```python
from build123d import *

# Parameters (mm, degrees)
F0_R     = 1.6
F0_W     = 21
F0_H     = 55
F1_DEPTH = 15
F2_W     = 22.6258952171
F2_H     = 57.1813471615
F3_DEPTH = 1
F5_DEPTH = 2
F6_SIZE  = 1.99999


# Not quite as in the source:
# - a fillet or chamfer is up to 0.001 mm smaller than in the source, because OpenCascade refuses the exact size


with BuildPart() as f1:
    # F0 (on Top) → F1 (new body)
    with BuildSketch(Plane.XY):
        with BuildLine():
            Line((12.5, -29.5), (12.5, 29.5))
            ThreePointArc((12.5, 29.5), (0, 42), (-12.5, 29.5))
            Line((-12.5, 29.5), (-12.5, -29.5))
            ThreePointArc((-12.5, -29.5), (0, -42), (12.5, -29.5))
        make_face()
        with Locations((-6, -33.5)):
            Circle(F0_R, mode=Mode.SUBTRACT)
        with Locations((6, -33.5)):
            Circle(F0_R, mode=Mode.SUBTRACT)
        with Locations((-6, 33.5)):
            Circle(F0_R, mode=Mode.SUBTRACT)
        Rectangle(F0_W, F0_H, mode=Mode.SUBTRACT)
        with Locations((6, 33.5)):
            Circle(F0_R, mode=Mode.SUBTRACT)
    extrude(amount=F1_DEPTH)

    # F2 (on Top) → F3 (join)
    with BuildSketch(Plane.XY):
        Rectangle(F2_W, F2_H)
    extrude(amount=F3_DEPTH)

    # F4 (on face) → F5 (cut)
    with BuildSketch(Plane.XY.offset(15)):
        with BuildLine():
            ThreePointArc((1.5, 41.909673646), (0, 42), (-1.5, 41.909673646))
            Line((-1.5, 41.909673646), (-1.5, 27.5))
            Line((-1.5, 27.5), (1.5, 27.5))
            Line((1.5, 27.5), (1.5, 41.909673646))
        make_face()
        with BuildLine():
            Line((1.5, -27.5), (-1.5, -27.5))
            Line((-1.5, -27.5), (-1.5, -41.909673646))
            ThreePointArc((-1.5, -41.909673646), (0, -42), (1.5, -41.909673646))
            Line((1.5, -41.909673646), (1.5, -27.5))
        make_face()
    extrude(amount=-F5_DEPTH, mode=Mode.SUBTRACT)

    # F6 (size 2 in the source; OpenCascade refuses exactly that, so slightly less here)
    f6_edges = [f1.edges().sort_by_distance(p)[0] for p in [
        (-1.5, 34.704837, 15),
        (1.5, 34.704837, 15),
        (1.5, -34.704837, 15),
        (-1.5, -34.704837, 15),
    ]]
    chamfer(f6_edges, length=F6_SIZE)


solid = f1.part
```
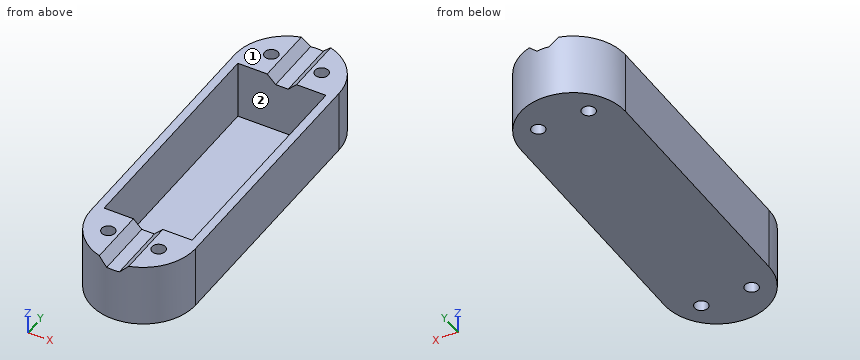
Check sheet for the modelled part. Datum: model origin and axes. Units: mm. Face numbers are marked on the shaded views. A direction names the side the tool comes from. Coordinates: 2 decimals unless noted, no trailing zeros. Order: outer loops, then holes, each group sorted by start corner. A loop starts at its lowest first (then second) coordinate and runs counter-clockwise, first axis right, second up. Notation, with made-up numbers: M 16,66 L 51,66 A17 cw 51,93 Z; hole C 24.5,83.5 d7. An arc over 180 degrees is marked long. One line per question, with ' | ' between items. Start each with the question number.
Item 1: Access from +Z, -Z, +X, -X, +Y, -Y to the whole of each face (thin tool, end or side, straight path). Record for the marked faces 1 and 2.
Item 2: Sectioned sample at D-D on x = -6. Record the cut outline in (y, z), and give its area (3 significant figures).
Item 3: Sectioned sample at A-A on z = 14. Record the cut outline in (x, y), and give its area (3 significant figures).
Item 4: Sectioned sample at C-C on y = 17. Record the cut outline in (x, z), and give its area (3 significant figures).
Item 5: Sectioned sample at B-B on z = 5. Record the cut outline in (x, y).
Item 6: Gauge pin test, flat ends, axial feed: P1, Ø1.5, axis at x = -0.5, y = 38, coming from the +Z side; P2, Ø5, axis at x = 6, z = 5.5, coming from the -Y side; P3, Ø3, axis at x = 9, z = 5, coming from the +Y side. Record the tip position at first contact, or that the pin passes through.
Item 7: Material ranges on line 1 (Y direction, x = -5.25, z = 6.25); line 2 (X direction, y = 12, z = 12.75); line 3 (Y direction, x = -6, z = 12.25), recorded low to high.
Answer below:
1) face 1: +Z, +X, -X, +Y, -Y | face 2: +Z
2) outline: M -40.47,0 L -35.1,0 L -35.1,15 L -40.47,15 Z; M -31.9,0 L 31.9,0 L 31.9,15 L 27.5,15 L 27.5,1 L -27.5,1 L -27.5,15 L -31.9,15 Z; M 35.1,0 L 40.47,0 L 40.47,15 L 35.1,15 Z | area: 348 mm^2
3) outline: M -12.5,-29.5 A12.5 ccw -2.5,-41.75 L -2.5,-27.5 L -10.5,-27.5 L -10.5,27.5 L -2.5,27.5 L -2.5,41.75 A12.5 ccw -12.5,29.5 Z; M 2.5,-41.75 A12.5 ccw 12.5,-29.5 L 12.5,29.5 A12.5 ccw 2.5,41.75 L 2.5,27.5 L 10.5,27.5 L 10.5,-27.5 L 2.5,-27.5 Z; hole C -6,-33.5 d3.2; hole C -6,33.5 d3.2; hole C 6,-33.5 d3.2; hole C 6,33.5 d3.2 | area: 635 mm^2
4) outline: M -12.5,0 L 12.5,0 L 12.5,15 L 10.5,15 L 10.5,1 L -10.5,1 L -10.5,15 L -12.5,15 Z | area: 81.0 mm^2
5) outline: M -12.5,-29.5 A12.5 ccw 12.5,-29.5 L 12.5,29.5 A12.5 ccw -12.5,29.5 Z; hole M -10.5,-27.5 L 10.5,-27.5 L 10.5,27.5 L -10.5,27.5 Z; hole C -6,-33.5 d3.2; hole C -6,33.5 d3.2; hole C 6,-33.5 d3.2; hole C 6,33.5 d3.2
6) P1: stops at z = 13 | P2: stops at y = -41.5 | P3: stops at y = 39.5
7) line 1: y = -40.84 to -34.91, -32.09 to -27.5, 27.5 to 32.09, 34.91 to 40.84 | line 2: x = -12.5 to -10.5, 10.5 to 12.5 | line 3: y = -40.47 to -35.1, -31.9 to -27.5, 27.5 to 31.9, 35.1 to 40.47
